The figure shows three views and two pictorial views of one solid part (mm, origin at its lowest corner). Answer the questions. Give positions to 0.01 mm unless a question says otherwise; leave off trailing zeros. Loops run counter-clockwise (first coordinate to the right, second up) from the corner with the lowest first, then second, coordinate; pieces in that order, holes last.
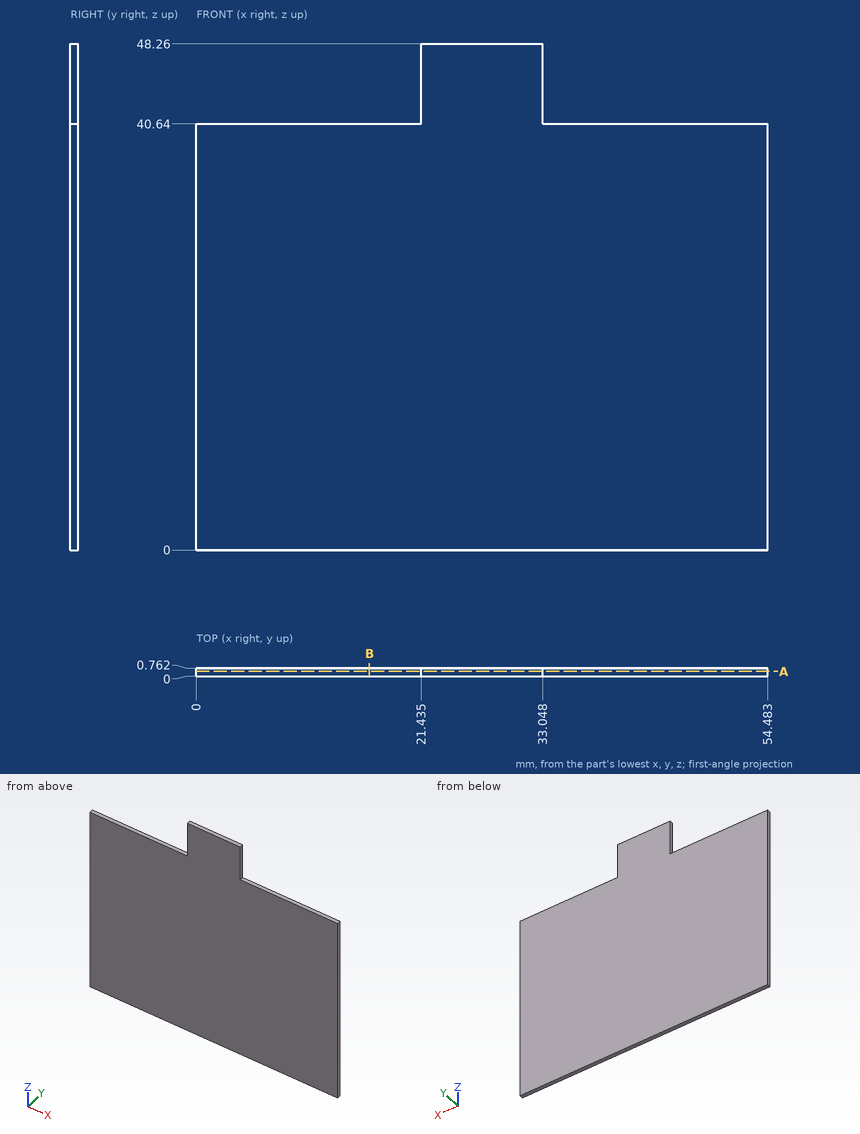
Q1. Consider line 1 along Z through (x, y) = (47, 0.05); line 2 along X through (y, z) = (0.5, 41) (1 decimal). Determine where each line is inside the solid, lowest interval first.
Q2. Given pin 1 (8 mm diameter, centred on x = 36, z = 22, fed in from -Y), flat-ended and moving along its own axis, determine where the tip first touches the part or whether it passes through.
Q3. Section A-A on y = 0.45 is taken. Give the vertices of the cut face in (x, z) (1 decimal), plus the area to 3 significant figures.
Q4. Section B-B on x = 16.5 is taken. Give the vertices of the cut face in (y, z).
Check result:
1. line 1: z = 0 to 40.64
1. line 2: x = 21.4 to 33
2. pin 1: stops at y = 0
3. outline: (0, 0) - (54.5, 0) - (54.5, 40.6) - (33, 40.6) - (33, 48.3) - (21.4, 48.3) - (21.4, 40.6) - (0, 40.6) - close
3. area: 2,300 mm2
4. outline: (0, 0) - (0.76, 0) - (0.76, 40.64) - (0, 40.64) - close
